from build123d import *

# Parameters (mm, degrees)
F0_W     = 98.895595
F0_H     = 99.196188
F0_W_2   = 42
F0_H_2   = 20
F0_R     = 10
F1_DEPTH = 100
F3_DEPTH = 25


with BuildPart() as f1:
    # F0 (on Front) → F1 (new body)
    with BuildSketch(Plane.XZ):
        Polygon((52.307254, -49.542874), (52.307254, 50.024388), (-47.259618, 50.024388), (-47.259618, 49.653314), (51.635977, 49.653314), (51.635977, -49.542874), align=None)
        with Locations((2.18818, 0.05522)):
            Rectangle(F0_W, F0_H)
        with Locations((0.514312, -34.132177)):
            Rectangle(F0_W_2, F0_H_2, mode=Mode.SUBTRACT)
        Polygon((5.228865, 0), (-5.271107, 0.024388), (0, 9.105436), align=None, mode=Mode.SUBTRACT)
        with Locations((-17.692746, 30.024388)):
            Circle(F0_R, mode=Mode.SUBTRACT)
        with Locations((22.307254, 30.024388)):
            Circle(F0_R, mode=Mode.SUBTRACT)
    extrude(amount=F1_DEPTH)

    # F0 (on Front) → F3 (join)
    with BuildSketch(Plane.XZ):
        Polygon((52.307254, -49.542874), (52.307254, 50.024388), (-47.259618, 50.024388), (-47.259618, 49.653314), (51.635977, 49.653314), (51.635977, -49.542874), align=None)
        with Locations((2.18818, 0.05522)):
            Rectangle(F0_W, F0_H)
        with Locations((0.514312, -34.132177)):
            Rectangle(F0_W_2, F0_H_2, mode=Mode.SUBTRACT)
        Polygon((5.228865, 0), (-5.271107, 0.024388), (0, 9.105436), align=None, mode=Mode.SUBTRACT)
        with Locations((-17.692746, 30.024388)):
            Circle(F0_R, mode=Mode.SUBTRACT)
        with Locations((22.307254, 30.024388)):
            Circle(F0_R, mode=Mode.SUBTRACT)
    extrude(amount=F3_DEPTH)


solid = f1.part
Geometry: final body of the model. Coordinates: model frame, mm. A direction names the side the tool comes from. Give positions to 0.01 mm unless a question says otherwise; leave off trailing zeros. Write each loop counter-clockwise with the first axis right and the second up, starting at its lowest first coordinate (ties: lowest second). Pieces come first, ordered by that corner, then holes. Notation, with made-up numbers: (-17, -31) -> (14, -31) arc R24 ccw to (14, -4) -> close; hole circle Ø9 at (9.5, -19.75). An arc over 180 degrees is marked (long way). Answer as a JSON object with one key per item and string values.
1. Ray query, probe 1 along Z at (x, y) = (3.5, -13.5); probe 2 along Z at (x, y) = (-15, -8); probe 3 along X at (y, z) = (-74, 25). Return the intervals inside material, ascending. Write a range as from..to.
Ans:
{"probe 1": "z = -49.54..-44.13, -24.13..0, 3.01..50.02", "probe 2": "z = -49.54..-44.13, -24.13..20.39, 39.66..50.02", "probe 3": "x = -47.26..-26.34, -9.05..13.66, 30.95..52.31"}
2. Cut plane B-B on x = 29.5. Output: boundary loops of the cut face in (y, z), and give its area (3 significant figures).
Ans:
{"outline": "(-100, -49.54) -> (0, -49.54) -> (0, 23.08) -> (-100, 23.08) -> close; (-100, 36.97) -> (0, 36.97) -> (0, 50.02) -> (-100, 50.02) -> close", "area": "8,570 mm^2"}
3. Contact query for a flat-ended pin moving along its axis: pin 1 (16 mm diameter, centred on x = -17.69, z = 30.02, fed in from +Y). Output: stop coordinate, or through.
Ans:
{"pin 1": "passes through"}
4. Cut plane A-A on z = -31. Output: boundary loops of the cut face in (x, y).
Ans:
{"outline": "(-47.26, -100) -> (-20.49, -100) -> (-20.49, 0) -> (-47.26, 0) -> close; (21.51, -100) -> (52.31, -100) -> (52.31, 0) -> (21.51, 0) -> close"}
5. Cut plane C-C on y = -92.5. Output: boundary loops of the cut face in (x, z).
Ans:
{"outline": "(-47.26, -49.54) -> (52.31, -49.54) -> (52.31, 50.02) -> (-47.26, 50.02) -> close; hole circle Ø20 at (-17.69, 30.02); hole (-20.49, -44.13) -> (21.51, -44.13) -> (21.51, -24.13) -> (-20.49, -24.13) -> close; hole (-5.27, 0.02) -> (5.23, 0) -> (0, 9.11) -> close; hole circle Ø20 at (22.31, 30.02)"}
6. Access query for faces 4 (the flat face through (3, -49, 50.024)), 5 (the flat face through (0, -49, -24.132)). Directions: +Z, -Z, +X, -X, +Y, -Y. A direction counts if a zero-diameter tool reaches every point of the face in a straight line with its end or side. Return the directions, or none.
Ans:
{"face 4": "+Z, +X, -X, +Y, -Y", "face 5": "+Y, -Y"}
7. Mould query, pull axis Z, two halves, no side actions, for faces 1 (the cylindrical face through (-12.32, -49.3, 38.46)), 2 (the flat face through (2, -49, -49.543)), 3 (the flat face through (-47.26, -49, -1)). Classes: pulls with the +Z half, pulls with the -Z half, needs draft (parallel to the pull), parting line crosses it, or undercut.
Ans:
{"face 1": "undercut", "face 2": "pulls with the -Z half", "face 3": "needs draft"}
